Geometry: final body of the model. Coordinates: model frame, mm. Face numbers are marked on the shaded views. Coordinates: 2 decimals unless noted, no trailing zeros. Order: outer loops, then holes, each group sorted by start corner. A loop starts at its lowest first (then second) coordinate and runs counter-clockwise, first axis right, second up. Notation, with made-up numbers: (50.5, -5) - (84.5, -5) arc R25 ccw to (84.5, 20) - close; hole circle Ø2 at (34, 79). An arc over 180 degrees is marked (long way). Use a Markdown table: item, result. Add a question column.
```python
from build123d import *

# Parameters (mm, degrees)
SKETCH1_R           = 2.15
BOSS_EXTRUDE1_DEPTH = 25.4
SKETCH2_R           = 27.5
CUT_EXTRUDE1_DEPTH  = 2.54


with BuildPart() as part:
    # Sketch1 → Boss-Extrude1 (new body)
    with BuildSketch(Plane.XY):
        with BuildLine():
            Line((25.000000038, 30), (-25.000000038, 30))
            ThreePointArc((-25.000000038, 30), (-28.535533911, 28.535533885), (-30, 25))
            Line((-30, 25), (-30, -25))
            ThreePointArc((-30, -25), (-28.535533911, -28.535533885), (-25.000000038, -30))
            Line((-25.000000038, -30), (25.000000038, -30))
            ThreePointArc((25.000000038, -30), (28.535533944, -28.535533906), (30.000000038, -25))
            Line((30, -25), (30, 25))
            ThreePointArc((30, 25), (28.535533911, 28.535533885), (25.000000038, 30))
        make_face()
        with Locations((-25.000000038, -25)):
            Circle(SKETCH1_R, mode=Mode.SUBTRACT)
        with Locations((25.000000038, -25)):
            Circle(SKETCH1_R, mode=Mode.SUBTRACT)
        with Locations((-25.000000038, 25)):
            Circle(SKETCH1_R, mode=Mode.SUBTRACT)
        with Locations((25.000000038, 25)):
            Circle(SKETCH1_R, mode=Mode.SUBTRACT)
    extrude(amount=BOSS_EXTRUDE1_DEPTH)

    # Sketch2 → Cut-Extrude1 (cut)
    with BuildSketch(Plane.XY.offset(25.4)):
        Circle(SKETCH2_R)
    extrude(amount=-CUT_EXTRUDE1_DEPTH, mode=Mode.SUBTRACT)


solid = part.part
```
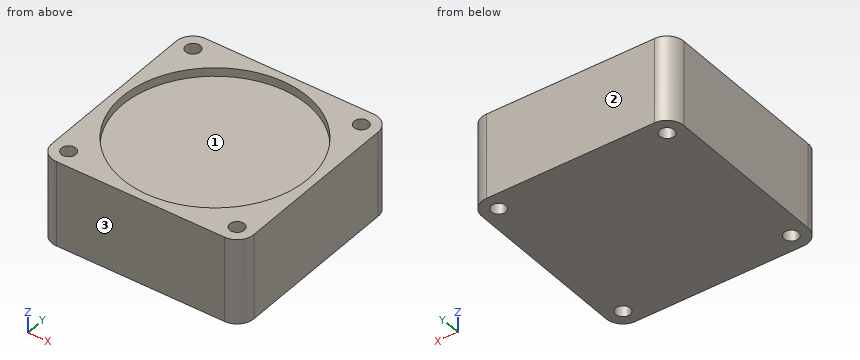
1) Ray query, line 1 along Y through (x, z) = (-25, 8.5); line 2 along Y through (x, z) = (26, 18.25); line 3 along Z through (x, y) = (-15, -18). Return the intervals inside material, ascending.
2) Draft query along Y for the marked faces 1, 2 and 3. Return one class per face: pulls with the +Y half, pulls with the -Y half, needs draft (parallel to the pull), parting line crosses it, or undercut.
3) Pin query (flat end, axial travel): pin 1 (1 mm diameter, centred on x = -13.5, y = 11.5, fed in from +Z). Return the tip coordinate at first contact, or that it passes through.
4) Section B-B (y = 0). Return loops of the section in (x, z).
5) Section A-A (x = 11.5). Return loops of the section in (y, z).
6) Section C-C (z = 15). Return loops of the section in (x, y), then the cut area to 3 significant figures.
Values follow:
| question | item | result |
|---|---|---|
| 1 | line 1 | y = -30 to -27.15, -22.85 to 22.85, 27.15 to 30 |
| 1 | line 2 | y = -29.9 to -26.9, -23.1 to 23.1, 26.9 to 29.9 |
| 1 | line 3 | z = 0 to 22.86 |
| 2 | face 1 | undercut |
| 2 | face 2 | pulls with the +Y half |
| 2 | face 3 | pulls with the -Y half |
| 3 | pin 1 | stops at z = 22.86 |
| 4 | outline | (-30, 0) - (30, 0) - (30, 25.4) - (27.5, 25.4) - (27.5, 22.86) - (-27.5, 22.86) - (-27.5, 25.4) - (-30, 25.4) - close |
| 5 | outline | (-30, 0) - (30, 0) - (30, 25.4) - (24.98, 25.4) - (24.98, 22.86) - (-24.98, 22.86) - (-24.98, 25.4) - (-30, 25.4) - close |
| 6 | outline | (-30, -25) arc R5 ccw to (-25, -30) - (25, -30) arc R5 ccw to (30, -25) - (30, 25) arc R5 ccw to (25, 30) - (-25, 30) arc R5 ccw to (-30, 25) - close; hole circle Ø4.3 at (-25, -25); hole circle Ø4.3 at (-25, 25); hole circle Ø4.3 at (25, -25); hole circle Ø4.3 at (25, 25) |
| 6 | area | 3,520 mm² |
